Here's the drawing with two shaded views (mm, measured from the low corner). I have some questions. Round coordinates to 2 decimals unless told otherwise and drop trailing zeros. Write each loop counter-clockwise with the first axis right and the second up, starting at its lowest first coordinate (ties: lowest second). Pieces come first, ordered by that corner, then holes. Notation, with made-up numbers: M 61.5,33.25 L 80.5,33.25 A33 ccw 80.5,66.25 Z; hole C 31,-29.75 d3. An arc over 180 degrees is marked long. Write item = value, one per line. Start each with the question number.
(1) I want a section at B-B (z = 9). List the corners of the cut face in (x, y) for me.
(2) Will this pin go through, and if not, where does the flat tip stop? pin 1 Ø5 at (x, z) = (25.5, 13) entering from -Y.
(3) I want a section at D-D (z = 3.25). List the corners of the cut face in (x, y) for me.
(4) I want a section at C-C (y = 4). List the corners of the cut face in (x, z) for me, and give its area (3 significant figures).
(5) If we mould it in two halves opening along Z, with no side actions, what happens to the marked faces 1, 2, 3 and 4? For each: released by +Z, released by -Z, zero draft, split by the parting line, or undercut.
(6) I want a section at A-A (x = 45). List the corners of the cut face in (y, z) for me.
(7) I need wall thicknesses on line 1 along Z through (x, y) = (74, 6.25); line 2 along X through (y, z) = (4.5, 1.25); line 3 along X through (y, z) = (5.25, 2.75). Which ranges of each line are inside material? Lowest first, please.
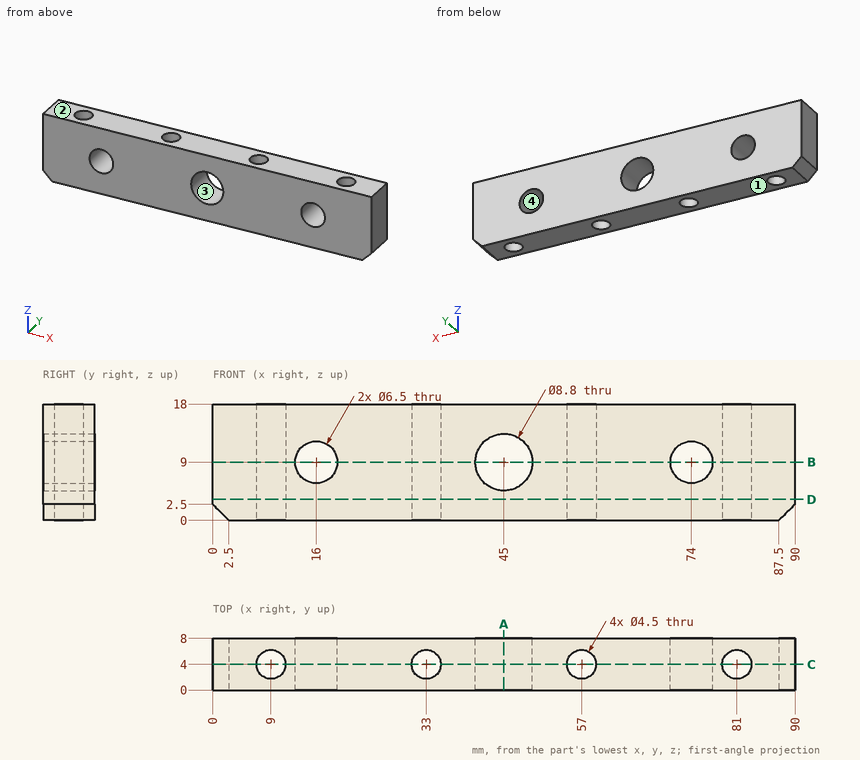
Returned:
q1.outline = M 0,0 L 12.75,0 L 12.75,8 L 0,8 Z; M 19.25,0 L 40.6,0 L 40.6,8 L 19.25,8 Z; M 49.4,0 L 70.75,0 L 70.75,8 L 49.4,8 Z; M 77.25,0 L 90,0 L 90,8 L 77.25,8 Z; hole C 9,4 d4.5; hole C 33,4 d4.5; hole C 57,4 d4.5; hole C 81,4 d4.5
q2.pin_1 = 0
q3.outline = M 0,0 L 90,0 L 90,8 L 0,8 Z; hole C 9,4 d4.5; hole C 33,4 d4.5; hole C 57,4 d4.5; hole C 81,4 d4.5
q4.outline = M 0,2.5 L 2.5,0 L 6.75,0 L 6.75,18 L 0,18 Z; M 11.25,0 L 30.75,0 L 30.75,18 L 11.25,18 Z; M 35.25,0 L 54.75,0 L 54.75,18 L 35.25,18 Z; M 59.25,0 L 78.75,0 L 78.75,18 L 59.25,18 Z; M 83.25,0 L 87.5,0 L 90,2.5 L 90,18 L 83.25,18 Z; hole C 16,9 d6.5; hole C 45,9 d8.8; hole C 74,9 d6.5
q4.area = 1,160 mm²
q5.face_1 = released by -Z
q5.face_2 = released by +Z
q5.face_3 = undercut
q5.face_4 = undercut
q6.outline = M 0,0 L 8,0 L 8,4.6 L 0,4.6 Z; M 0,13.4 L 8,13.4 L 8,18 L 0,18 Z
q7.line_1 = 0 to 5.75, 12.25 to 18
q7.line_2 = 1.25 to 6.81, 11.19 to 30.81, 35.19 to 54.81, 59.19 to 78.81, 83.19 to 88.75
q7.line_3 = 0 to 7.13, 10.87 to 31.13, 34.87 to 55.13, 58.87 to 79.13, 82.87 to 90
